from build123d import *

# Parameters (mm, degrees)
BOSS_EXTRUDE1_DEPTH = 1
SKETCH2_W           = 3.399574798
SKETCH2_H           = 2.604207363
SKETCH2_W_2         = 0.648007004
SKETCH2_H_2         = 1.252018983
BOSS_EXTRUDE2_DEPTH = 0.5
SKETCH3_W           = 2.913906285
SKETCH3_H           = 1.803051724
CUT_EXTRUDE1_DEPTH  = 1
SKETCH4_W           = 0.755256807
SKETCH4_H           = 1.639917717
SKETCH4_W_2         = 0.763724631
SKETCH4_H_2         = 1.626197377
BOSS_EXTRUDE3_DEPTH = 1
SKETCH6_W           = 0.323055787
SKETCH6_H           = 1.224923668
SKETCH6_W_2         = 0.371772392
SKETCH6_H_2         = 1.735099538
SKETCH6_W_3         = 0.361493721
SKETCH6_H_3         = 2.070814397
BOSS_EXTRUDE4_DEPTH = 0.3
BOSS_EXTRUDE8_DEPTH = 0.3


with BuildPart() as part:
    # Sketch1 → Boss-Extrude1 (new body)
    with BuildSketch(Plane(origin=(0, 0, 0), x_dir=(1, 0, 0), z_dir=(0, 1, 0))):
        with BuildLine():
            Line((-8.75, 20.5), (8.75, 20.5))
            ThreePointArc((8.75, 20.5), (14.406854249, 18.156854249), (16.75, 12.5))
            Line((16.75, 12.5), (16.75, -12.5))
            ThreePointArc((16.75, -12.5), (14.406854249, -18.156854249), (8.75, -20.5))
            Line((8.75, -20.5), (-8.75, -20.5))
            ThreePointArc((-8.75, -20.5), (-14.406854249, -18.156854249), (-16.75, -12.5))
            Line((-16.75, -12.5), (-16.75, 12.5))
            ThreePointArc((-16.75, 12.5), (-14.406854249, 18.156854249), (-8.75, 20.5))
        make_face()
    extrude(amount=BOSS_EXTRUDE1_DEPTH)

    # Sketch2 → Boss-Extrude2 (add)
    with BuildSketch(Plane(origin=(0, 1, 0), x_dir=(1, 0, 0), z_dir=(0, 1, 0))):
        with Locations((-10.250837729, 15.647459094)):
            Rectangle(SKETCH2_W, SKETCH2_H)
        with Locations((-12.27462863, 15.762007905)):
            Rectangle(SKETCH2_W_2, SKETCH2_H_2)
    extrude(amount=BOSS_EXTRUDE2_DEPTH)

    # Sketch3 → Cut-Extrude1 (cut)
    with BuildSketch(Plane(origin=(0, 1.5, 0), x_dir=(1, 0, 0), z_dir=(0, 1, 0))):
        with Locations((-10.221842574, 15.632123632)):
            Rectangle(SKETCH3_W, SKETCH3_H)
    extrude(amount=-CUT_EXTRUDE1_DEPTH, mode=Mode.SUBTRACT)

    # Sketch4 → Boss-Extrude3 (add)
    with BuildSketch(Plane(origin=(0, 0.5, 0), x_dir=(1, 0, 0), z_dir=(0, 1, 0))):
        with Locations((-9.510068413, 15.646512941)):
            Rectangle(SKETCH4_W, SKETCH4_H)
        with Locations((-10.421480669, 15.658650775)):
            Rectangle(SKETCH4_W_2, SKETCH4_H_2)
    extrude(amount=BOSS_EXTRUDE3_DEPTH)

    # Sketch6 → Boss-Extrude4 (add)
    with BuildSketch(Plane(origin=(0, 1, 0), x_dir=(1, 0, 0), z_dir=(0, 1, 0))):
        with Locations((-7.401507334, 15.079514795)):
            Rectangle(SKETCH6_W, SKETCH6_H)
        with Locations((-6.585633976, 15.340608205)):
            Rectangle(SKETCH6_W_2, SKETCH6_H_2)
        with Locations((-5.759844772, 15.498462338)):
            Rectangle(SKETCH6_W_3, SKETCH6_H_3)
    extrude(amount=BOSS_EXTRUDE4_DEPTH)

    # Sketch7 → Boss-Extrude8 (add)
    with BuildSketch(Plane(origin=(0, 1, 0), x_dir=(1, 0, 0), z_dir=(0, 1, 0))):
        Polygon((-2.913348429, 17.083305865), (-3.070822573, 16.069437014), (-3.890044364, 16.734757778), (-4.10463288, 16.470530961), (-3.125803438, 15.71545264), (-3.128811108, 15.696088298), (-4.220670364, 15.251854963), (-4.125911477, 15.018951756), (-3.168901436, 15.437973959), (-3.374102624, 14.116823145), (-1.801517614, 14.921145153), (-2.70763201, 15.653067043), (-1.594376902, 16.222457937), align=None)
        Polygon((-2.913348429, 15.389877589), (-3.025116607, 14.50250057), (-2.208716049, 14.94618908), align=None, mode=Mode.SUBTRACT)
        Polygon((-2.834687196, 15.935171595), (-2.70763201, 16.678238629), (-1.993867712, 16.306705112), align=None, mode=Mode.SUBTRACT)
    extrude(amount=BOSS_EXTRUDE8_DEPTH)


solid = part.part
Input: part model. Units: mm. Frame: model coordinates. A direction names the side the tool comes from. Coordinates: 2 decimals unless noted, no trailing zeros. Loops run counter-clockwise (first coordinate to the right, second up) from the corner with the lowest first, then second, coordinate; pieces in that order, holes last.
(1) Material intervals for probe 1 along Y at (x, z) = (-2, 9.5); probe 2 along X at (y, z) = (0.2, 18.5); probe 3 along X at (y, z) = (0.7, -13.5), sorted ascending.
(2) Section B-B on x = 4. Return the cut outline in (y, z).
(3) Section A-A on y = 0.25. Return the cut outline in (x, z), then the cut area to 3 significant figures.
(4) Section C-C on z = 9.5. Return the cut outline in (x, y), then the cut area to 3 significant figures.
(5) Set-up query: faces 4 (the face through (-2.9, 1.3, -15.7)), 5 (the face through (14.344, 0.493, -18.219)), 6 (the face through (-11, 1, -16.534)). Return all of +Z, -Z, +X, -X, +Y, -Y with unobstructed straight access to the full face (end or side cutting, diameter ignored); none if empty.
(6) Pull-direction query (X, two-part tool) for faces 1 (the face through (-10.04, 1, -16)), 2 (the face through (-16.75, 0.5, 0.2)), 3 (the face through (-0.1, 0.5, -20.5)); classes: released by +X, released by -X, zero draft, split by the parting line, or undercut.
(7) First-contact query: pin 1 Ø0.8 at (y, z) = (1, -15.5) entering from -X; pin 2 Ø0.5 at (y, z) = (1, -16) entering from -X; pin 3 Ø0.5 at (x, y) = (-9.5, 1) entering from -Z. Flat tips, straight axial feed; report the tip coordinate or a pass-through.
Data:
1. probe 1: y = 0 to 1
1. probe 2: x = -14.04 to 14.04
1. probe 3: x = -16.69 to 16.69
2. outline: (0, -20.5) - (1, -20.5) - (1, 20.5) - (0, 20.5) - close
3. outline: (-16.75, -12.5) arc R8 ccw to (-8.75, -20.5) - (8.75, -20.5) arc R8 ccw to (16.75, -12.5) - (16.75, 12.5) arc R8 ccw to (8.75, 20.5) - (-8.75, 20.5) arc R8 ccw to (-16.75, 12.5) - close
3. area: 1,320 mm2
4. outline: (-16.75, 0) - (16.75, 0) - (16.75, 1) - (-16.75, 1) - close
4. area: 33.5 mm2
5. face 4: +Z, -Z, +X, +Y
5. face 5: -Z, +X, +Y, -Y
5. face 6: +Y
6. face 1: undercut
6. face 2: released by -X
6. face 3: zero draft
7. pin 1: stops at x = -16.32
7. pin 2: stops at x = -16.06
7. pin 3: stops at z = -20.48
